from build123d import *

# Parameters (mm, degrees)
SKETCH_1_W          = 104.4
SKETCH_1_H          = 108.4
EXTRUDE_1_DEPTH     = 32.4
SKETCH_2_W          = 102
SKETCH_2_H          = 106
CUT_EXTRUDE_1_DEPTH = 31.2
EXTRUDE_2_DEPTH     = 10
SKETCH_6_W          = 4
SKETCH_6_H          = 4
EXTRUDE_3_DEPTH     = 10
SKETCH_7_W          = 4
SKETCH_7_H          = 4
EXTRUDE_4_DEPTH     = 10
SKETCH_10_W         = 4
SKETCH_10_H         = 4
EXTRUDE_5_DEPTH     = 10


with BuildPart() as part:
    # 草图1 → 凸台-拉伸1 (new body)
    with BuildSketch(Plane(origin=(0, 0, 0), x_dir=(1, 0, 0), z_dir=(0, 1, 0))):
        Rectangle(SKETCH_1_W, SKETCH_1_H)
    extrude(amount=EXTRUDE_1_DEPTH)

    # 草图2 → 切除-拉伸1 (cut)
    with BuildSketch(Plane(origin=(0, 32.4, 0), x_dir=(1, 0, 0), z_dir=(0, 1, 0))):
        Rectangle(SKETCH_2_W, SKETCH_2_H)
    extrude(amount=-CUT_EXTRUDE_1_DEPTH, mode=Mode.SUBTRACT)

    # 草图3 → 凸台-拉伸2 (add)
    with BuildSketch(Plane(origin=(0, 1.2, 0), x_dir=(1, 0, 0), z_dir=(0, 1, 0))):
        Polygon((48, -53), (51, -53), (51, -52.54057914), (51, -50), (48, -50), align=None)
    extrude(amount=EXTRUDE_2_DEPTH)

    # 草图6 → 凸台-拉伸3 (add)
    with BuildSketch(Plane(origin=(0, 1.2, 0), x_dir=(1, 0, 0), z_dir=(0, 1, 0))):
        with Locations((49, 51)):
            Rectangle(SKETCH_6_W, SKETCH_6_H)
    extrude(amount=EXTRUDE_3_DEPTH)

    # 草图7 → 凸台-拉伸4 (add)
    with BuildSketch(Plane(origin=(0, 1.2, 0), x_dir=(1, 0, 0), z_dir=(0, 1, 0))):
        with Locations((-49, -51)):
            Rectangle(SKETCH_7_W, SKETCH_7_H)
    extrude(amount=EXTRUDE_4_DEPTH)

    # 草图10 → 凸台-拉伸5 (add)
    with BuildSketch(Plane(origin=(0, 1.2, 0), x_dir=(1, 0, 0), z_dir=(0, 1, 0))):
        with Locations((-49, 50.130572063)):
            Rectangle(SKETCH_10_W, SKETCH_10_H)
    extrude(amount=EXTRUDE_5_DEPTH)


solid = part.part
Work out the finished part from the listing and answer in its coordinate system (mm). A direction names the side the tool comes from. Give positions to 0.01 mm unless a question says otherwise; leave off trailing zeros. Order: outer loops, then holes, each group sorted by start corner. A loop starts at its lowest first (then second) coordinate and runs counter-clockwise, first axis right, second up. Notation, with made-up numbers: (-12.75, 28) - (11.25, 28) arc R32 cw to (11.25, 57) - close; hole circle Ø4 at (87.25, 3). An arc over 180 degrees is marked (long way). Answer as CSV lines item,"result". Start each with the question number.
Q1. The mould has two halves that part along Z. Classify faces 1 (the face through (-1, 0, -1)), 2 (the face through (-49, 11.2, 51)), 3 (the face through (-1, 16, 54.2)): +Z half, -Z half, draft (parallel to the pull), parting line (faces both ways), or undercut.
Q2. The part is cut by section C-C (z = 45). Write down the section's boundary in (x, y), then the cut area to 3 significant figures.
Q3. Find the intervals of material crossed by L1, parallel to Z at x = 35, y = 16.5; L2, parallel to X at y = 4, z = -12.5; L3, parallel to Y at x = 31.5, z = -21, in increasing order. Write a range as [from, to].
Q4. The part is cut by section B-B (x = 44.5). Write down the section's boundary in (y, z), then the cut area to 3 significant figures.
Q5. Given pin 1 Ø5 at (x, z) = (4.5, 2) entering from +Y, flat-ended and moving along its own axis, determine where the tip first touches the part or whether it passes through.
Q6. For faces 4 (the face through (-52.2, 16, 1)), 5 (the face through (48, 6, 51)), determine the directions among +Z, -Z, +X, -X, +Y, -Y from which every point of the face is accessible in a straight line to the end or side of a thin tool.
Q7. The part is cut by section D-D (y = 26.5). Write down the section's boundary in (x, z), then the cut area to 3 significant figures.
Q8. The part is cut by section A-A (y = 5). Write down the section's boundary in (x, z), then the cut area to 3 significant figures.
Check result:
1,face 1,"draft"
1,face 2,"undercut"
1,face 3,"+Z half"
2,outline,"(-52.2, 0) - (52.2, 0) - (52.2, 32.4) - (51, 32.4) - (51, 1.2) - (-51, 1.2) - (-51, 32.4) - (-52.2, 32.4) - close"
2,area,"200 mm²"
3,L1,"z = [-54.2, -53], [53, 54.2]"
3,L2,"x = [-52.2, -51], [51, 52.2]"
3,L3,"y = [0, 1.2]"
4,outline,"(0, -54.2) - (32.4, -54.2) - (32.4, -53) - (1.2, -53) - (1.2, 53) - (32.4, 53) - (32.4, 54.2) - (0, 54.2) - close"
4,area,"205 mm²"
5,pin 1,"stops at y = 1.2"
6,face 4,"+Z, -Z, -X, +Y, -Y"
6,face 5,"+Y"
7,outline,"(-52.2, -54.2) - (52.2, -54.2) - (52.2, 54.2) - (-52.2, 54.2) - close; hole (-51, -53) - (51, -53) - (51, 53) - (-51, 53) - close"
7,area,"505 mm²"
8,outline,"(-52.2, -54.2) - (52.2, -54.2) - (52.2, 54.2) - (-52.2, 54.2) - close; hole (-51, -53) - (47, -53) - (47, -49) - (51, -49) - (51, 50) - (48, 50) - (48, 53) - (-47, 53) - (-47, 49) - (-51, 49) - (-51, -48.13) - (-47, -48.13) - (-47, -52.13) - (-51, -52.13) - close"
8,area,"562 mm²"
